Geometry: final body of the model. Coordinates: model frame, mm. Coordinates: 2 decimals unless noted, no trailing zeros. Write each loop counter-clockwise with the first axis right and the second up, starting at its lowest first coordinate (ties: lowest second). Pieces come first, ordered by that corner, then holes.
from build123d import *

# Parameters (mm, degrees)
F1_DEPTH = 38.1


with BuildPart() as f1:
    # F0 (on Right) → F1 (new body)
    with BuildSketch(Plane.YZ):
        with BuildLine():
            Line((-114.3, 0), (0, -20.154174))
            Line((0, -20.154174), (0, 139.7))
            ThreePointArc((0, 139.7), (-25.4, 196.496127), (0, 253.292253))
            Line((0, 253.292253), (0, 292.1))
            Line((0, 292.1), (-114.3, 312.254174))
            Line((-114.3, 312.254174), (-114.3, 253.292253))
            ThreePointArc((-114.3, 253.292253), (-88.9, 196.496127), (-114.3, 139.7))
            Line((-114.3, 139.7), (-114.3, 0))
        make_face()
    extrude(amount=F1_DEPTH)


solid = f1.part
Item 1: Section C-C, the plane z = 147. Output: boundary loops of the cut face in (x, y), plus the area to 3 significant figures.
Derived:
outline: (0, -107.16) - (38.1, -107.16) - (38.1, -7.14) - (0, -7.14) - close
area: 3,810 mm2
Item 2: Section D-D, the plane y = -55. Output: boundary loops of the cut face in (x, z), plus the area to 3 significant figures.
Derived:
outline: (0, -10.46) - (38.1, -10.46) - (38.1, 301.8) - (0, 301.8) - close
area: 11,900 mm2
Item 3: Pin query (flat end, axial travel): pin 1 (1 mm diameter, centred on x = 18, y = -100, fed in from +Z); pin 2 (1.5 mm diameter, centred on x = 17, z = 173, fed in from +Y). Return the tip coordinate at first contact, or that it passes through.
Derived:
pin 1: stops at z = 309.82
pin 2: stops at y = -21.44
Item 4: Section A-A, the plane y = -18.5. Output: boundary loops of the cut face in (x, z).
Derived:
outline: (0, -16.89) - (38.1, -16.89) - (38.1, 164.81) - (0, 164.81) - close; (0, 228.18) - (38.1, 228.18) - (38.1, 295.36) - (0, 295.36) - close
Item 5: Section B-B, the plane x = 11. Output: boundary loops of the cut face in (y, z).
Derived:
outline: (-114.3, 0) - (0, -20.15) - (0, 139.7) arc R76.2 cw to (0, 253.29) - (0, 292.1) - (-114.3, 312.25) - (-114.3, 253.29) arc R76.2 cw to (-114.3, 139.7) - close
Item 6: Pull-direction query (Z, two-part tool) for faces 1 (the cylindrical face through (18.783, -25.395, 195.599)), 2 (the cylindrical face through (18.783, -88.905, 197.393)), 3 (the flat face through (18.783, -57.95, -9.936)), 4 (the flat face through (19, 0, 59)); classes: released by +Z, released by -Z, zero draft, split by the parting line, or undercut.
Derived:
face 1: undercut
face 2: undercut
face 3: released by -Z
face 4: zero draft
Item 7: Material intervals for probe 1 along Z at (x, y) = (6.5, -15.5); probe 2 along Z at (x, y) = (7, -18); probe 3 along Z at (x, y) = (19.5, -68), sorted ascending.
Derived:
probe 1: z = -17.42 to 158.94, 234.06 to 294.83
probe 2: z = -16.98 to 163.74, 229.25 to 295.27
probe 3: z = -8.16 to 304.09
